Source: CAD feature listing. Evaluate the final solid. Frame: model axes, mm. A direction names the side the tool comes from. Give positions to 0.01 mm unless a question says otherwise; leave off trailing zeros. Order: outer loops, then holes, each group sorted by start corner. A loop starts at its lowest first (then second) coordinate and runs counter-clockwise, first axis right, second up. Notation, with made-up numbers: (-23.75, -24) -> (5.25, -24) arc R12 cw to (5.25, -19) -> close; hole circle Ø2 at (23.5, 34.5). An arc over 180 degrees is marked (long way). Answer in a Markdown table with one row per item.
```python
from build123d import *

# Parameters (mm, degrees)
F1_DEPTH = 22.86
F0_R     = 19.05
F2_DEPTH = 76.2
F3_DEPTH = 22.86
F0_W     = 106.68
F0_H     = 17.78
F4_DEPTH = 76.2
F6_DEPTH = 25.4


with BuildPart() as f1:
    # F0 (on Top) → F1 (new body)
    with BuildSketch(Plane.XY):
        Polygon((45.72, -8.450483), (45.72, -37.628572), (129.54, -37.660483), (152.4, -14.800483), (152.4, -8.450483), align=None)
    extrude(amount=F1_DEPTH)

    # F0 (on Top) → F2 (join)
    with BuildSketch(Plane.XY):
        with BuildLine():
            Line((45.72, 38.255124), (0, 38.1))
            ThreePointArc((0, 38.1), (-37.977013, 3.05884), (-6.097931, -37.608845))
            Line((-6.097931, -37.608845), (45.72, -37.628572))
            Line((45.72, -37.628572), (45.72, -8.450483))
            Line((45.72, -8.450483), (45.72, 9.329517))
            Line((45.72, 9.329517), (45.72, 38.255124))
        make_face()
        Circle(F0_R, mode=Mode.SUBTRACT)
    extrude(amount=F2_DEPTH)

    # F0 (on Top) → F3 (join)
    with BuildSketch(Plane.XY):
        Polygon((129.54, 38.539517), (45.72, 38.255124), (45.72, 9.329517), (152.4, 9.329517), (152.4, 15.679517), align=None)
    extrude(amount=F3_DEPTH)

    # F0 (on Top) → F4 (join)
    with BuildSketch(Plane.XY):
        with Locations((99.06, 0.439517)):
            Rectangle(F0_W, F0_H)
    extrude(amount=F4_DEPTH)

    # F5 (on face) → F6 (cut)
    with BuildSketch(Plane.XZ.offset(8.450483)):
        Polygon((152.4, 76.2), (45.72, 76.2), (152.4, 22.86), align=None)
    extrude(amount=-F6_DEPTH, mode=Mode.SUBTRACT)


solid = f1.part
```
(1) Section query A-A (y = 0). Return the cut outline in (x, z).
A:
| item | result |
|---|---|
| outline | (-38.1, 0) -> (-19.05, 0) -> (-19.05, 76.2) -> (-38.1, 76.2) -> close; (19.05, 0) -> (152.4, 0) -> (152.4, 22.86) -> (45.72, 76.2) -> (19.05, 76.2) -> close |
(2) Ray query, probe 1 along Y at (x, z) = (0, 53); probe 2 along X at (y, z) = (-1, 13); probe 3 along Y at (x, z) = (76.5, 42.5). Return the intervals inside material, ascending.
A:
| item | result |
|---|---|
| probe 1 | y = -37.61 to -19.05, 19.05 to 38.1 |
| probe 2 | x = -38.09 to -19.02, 19.02 to 152.4 |
| probe 3 | y = -8.45 to 9.33 |
(3) Section query D-D (z = 62.5). Return the cut outline in (x, y).
A:
| item | result |
|---|---|
| outline | (-6.1, -37.61) -> (45.72, -37.63) -> (45.72, -8.45) -> (73.12, -8.45) -> (73.12, 9.33) -> (45.72, 9.33) -> (45.72, 38.26) -> (0, 38.1) arc R38.1 ccw to start; hole circle Ø38.1 at (0, 0) |
(4) Access query for faces 1 (the flat face through (45.72, -23, 49)), 2 (the flat face through (98, 24, 22.86)), 3 (the flat face through (56, 1, 0)). Directions: +Z, -Z, +X, -X, +Y, -Y. A direction counts if a zero-diameter tool reaches every point of the face in a straight line with its end or side. Return the directions, or none.
A:
| item | result |
|---|---|
| face 1 | +Z, +X, -Y |
| face 2 | +Z, +X, +Y |
| face 3 | -Z, +X, -X, +Y, -Y |
(5) Section query C-C (x = 112). Return the cut outline in (y, z), plus the area to 3 significant figures.
A:
| item | result |
|---|---|
| outline | (-37.65, 0) -> (38.48, 0) -> (38.48, 22.86) -> (9.33, 22.86) -> (9.33, 43.06) -> (-8.45, 43.06) -> (-8.45, 22.86) -> (-37.65, 22.86) -> close |
| area | 2,100 mm^2 |
(6) Section query B-B (z = 39). Return the cut outline in (x, y).
A:
| item | result |
|---|---|
| outline | (-6.1, -37.61) -> (45.72, -37.63) -> (45.72, -8.45) -> (120.12, -8.45) -> (120.12, 9.33) -> (45.72, 9.33) -> (45.72, 38.26) -> (0, 38.1) arc R38.1 ccw to start; hole circle Ø38.1 at (0, 0) |
(7) First-contact query: pin 1 Ø6 at (y, z) = (-12, 59.5) entering from +X; pin 2 Ø4 at (x, y) = (78.5, 12.5) entering from +Z. Flat tips, straight axial feed; report the tip coordinate or a pass-through.
A:
| item | result |
|---|---|
| pin 1 | stops at x = 45.72 |
| pin 2 | stops at z = 22.86 |
(8) Pull-direction query (X, two-part tool) for faces 4 (the cylindrical face through (-15.12, -11.59, 37.57)), 5 (the flat face through (98, -23, 22.86)), 6 (the cylindrical face through (-37.9, 3.9, 37.6)), 7 (the flat face through (140.8, -26.4, 11.3)); classes: +X half, -X half, draft (parallel to the pull), parting line (faces both ways), or undercut.
A:
| item | result |
|---|---|
| face 4 | undercut |
| face 5 | draft |
| face 6 | -X half |
| face 7 | +X half |
